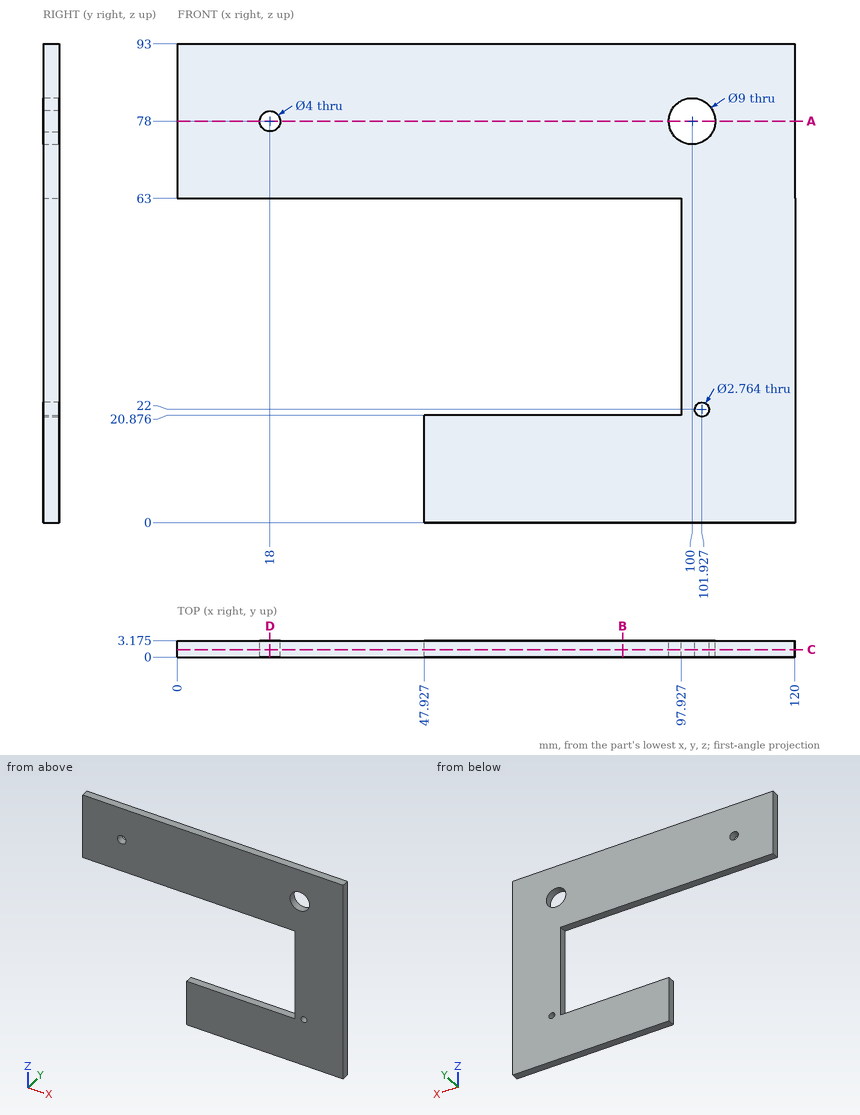
Drawing for the job (mm, zero at the part's lowest x, y, z). Give positions to 0.01 mm unless a question says otherwise; leave off trailing zeros. Write each loop counter-clockwise with the first axis right and the second up, starting at its lowest first coordinate (ties: lowest second). Pieces come first, ordered by that corner, then holes. Notation, with made-up numbers: (-31.75, 84.5) - (-10.75, 84.5) arc R23 ccw to (-10.75, 111.5) - close; hole circle Ø5 at (53.25, 75.25). An arc over 180 degrees is marked (long way). Answer as CSV lines item,"result".
Q1. Band-saw the part on C-C (y = 1.45). Give the cut face in (x, z).
Result set:
outline,"(0, 63) - (97.93, 63) - (97.93, 20.88) - (47.93, 20.88) - (47.93, 0) - (120, 0) - (120, 93) - (0, 93) - close; hole circle Ø4 at (18, 78); hole circle Ø9 at (100, 78); hole circle Ø2.76 at (101.93, 22)"
Q2. Drill centre lines: line 1 (X direction, y = 2.4, z = 78); line 2 (Z direction, x = 70, y = 2.75); line 3 (X direction, y = 1.45, z = 22) (1 decimal). Where is each one in solid material? Low to high. Write a range as from..to.
Result set:
line 1,"0..16, 20..95.5, 104.5..120"
line 2,"0..20.88, 63..93"
line 3,"97.9..100.5, 103.3..120"
Q3. Band-saw the part on B-B (x = 86.5). Give the cut face in (y, z) (1 decimal).
Result set:
outline,"(0, 0) - (3.2, 0) - (3.2, 20.9) - (0, 20.9) - close; (0, 63) - (3.2, 63) - (3.2, 93) - (0, 93) - close"
Q4. Flat gauge pins, fed straight in: pin 1 Ø1 at (y, z) = (1.5, 34.5) entering from -X; pin 2 Ø1.7 at (x, z) = (101.93, 22) entering from -Y; pin 3 Ø1.6 at (y, z) = (1.5, 7) entering from -X; pin 4 Ø1 at (x, y) = (43, 1.5) entering from -Z. Where does each tip first touch, or does it go through?
Result set:
pin 1,"x = 97.93"
pin 2,"through"
pin 3,"x = 47.93"
pin 4,"z = 63"
Q5. Band-saw the part on D-D (x = 18). Give the cut face in (y, z) (1 decimal).
Result set:
outline,"(0, 63) - (3.2, 63) - (3.2, 76) - (0, 76) - close; (0, 80) - (3.2, 80) - (3.2, 93) - (0, 93) - close"
Q6. Band-saw the part on A-A (z = 78). Give the cut face in (x, y) (1 decimal).
Result set:
outline,"(0, 0) - (16, 0) - (16, 3.2) - (0, 3.2) - close; (20, 0) - (95.5, 0) - (95.5, 3.2) - (20, 3.2) - close; (104.5, 0) - (120, 0) - (120, 3.2) - (104.5, 3.2) - close"
